Read the model definition and answer for the solid it produces. Units are mm, in the model's axes. Face numbers are marked on the shaded views. Give positions to 0.01 mm unless a question says otherwise; leave off trailing zeros. Order: outer loops, then holes, each group sorted by start corner. A loop starts at its lowest first (then second) coordinate and runs counter-clockwise, first axis right, second up. Notation, with made-up numbers: (-34, -36.5) -> (-8, -36.5) arc R18 cw to (-8, -5.5) -> close; hole circle Ø6 at (-30, -31.5). An arc over 180 degrees is marked (long way). One line per item, written item: value. Start each with the question number.
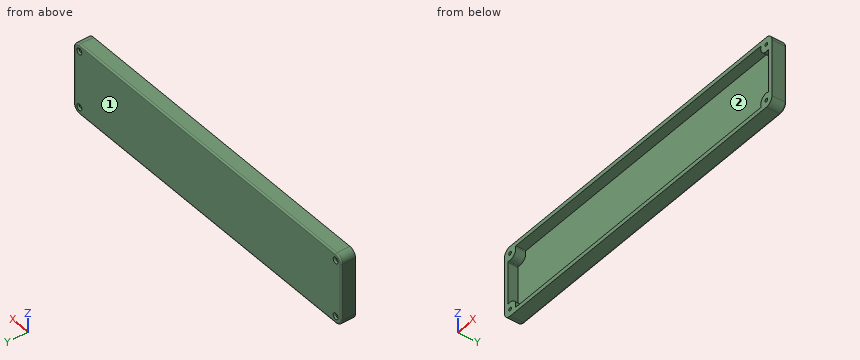
from build123d import *

# Parameters (mm, degrees)
BOSS_EXTRUDE1_DEPTH                                 = 10
CUT_EXTRUDE1_DEPTH                                  = 7
CSK_FOR_M2_COUNTERSUNK_FLAT_HEAD_SCREW2_D           = 2.4
CSK_FOR_M2_COUNTERSUNK_FLAT_HEAD_SCREW2_CSINK_D     = 4.4
CSK_FOR_M2_COUNTERSUNK_FLAT_HEAD_SCREW2_CSINK_ANGLE = 90
FILLET1_R                                           = 1


with BuildPart() as part:
    # Sketch1 → Boss-Extrude1 (new body)
    with BuildSketch(Plane(origin=(0, 0, 0), x_dir=(1, 0, 0), z_dir=(0, 1, 0))):
        with BuildLine():
            Line((-115, 25), (115, 25))
            ThreePointArc((115, 25), (118.535533906, 23.535533906), (120, 20))
            Line((120, 20), (120, -20))
            ThreePointArc((120, -20), (118.535533906, -23.535533906), (115, -25))
            Line((115, -25), (-115, -25))
            ThreePointArc((-115, -25), (-118.535533906, -23.535533906), (-120, -20))
            Line((-120, -20), (-120, 20))
            ThreePointArc((-120, 20), (-118.535533906, 23.535533906), (-115, 25))
        make_face()
    extrude(amount=-BOSS_EXTRUDE1_DEPTH)

    # Sketch2 → Cut-Extrude1 (cut)
    with BuildSketch(Plane.XZ.offset(10)):
        with BuildLine():
            ThreePointArc((110.125928985, 21.347074542), (111.23652041, 16.476032992), (115.978966674, 14.904516992))
            ThreePointArc((115.978966674, 14.904516992), (116.536912433, 15.216669336), (116.945654989, 14.725067791))
            Line((116.945654989, 14.725067791), (116.945654989, -14.725067791))
            ThreePointArc((116.945654989, -14.725067791), (116.58492435, -15.205280291), (116.023238809, -14.992583342))
            ThreePointArc((116.023238809, -14.992583342), (111.282334907, -16.506525423), (110.125928985, -21.347074542))
            ThreePointArc((110.125928985, -21.347074542), (110.043745309, -21.784949523), (109.644883292, -21.983438179))
            Line((109.644883292, -21.983438179), (-109.644883292, -21.983438179))
            ThreePointArc((-109.644883292, -21.983438179), (-110.043745309, -21.784949523), (-110.125928985, -21.347074542))
            ThreePointArc((-110.125928985, -21.347074542), (-111.42230579, -16.46889365), (-116.309291353, -15.206113484))
            ThreePointArc((-116.309291353, -15.206113484), (-116.747166334, -15.123929808), (-116.945654989, -14.725067791))
            Line((-116.945654989, -14.725067791), (-116.945654989, 14.725067791))
            ThreePointArc((-116.945654989, 14.725067791), (-116.746289712, 15.124590961), (-116.307179936, 15.205509941))
            ThreePointArc((-116.307179936, 15.205509941), (-111.411229141, 16.459961189), (-110.126182098, 21.347970622))
            ThreePointArc((-110.126182098, 21.347970622), (-110.043464387, 21.78532079), (-109.644883292, 21.983438179))
            Line((-109.644883292, 21.983438179), (109.644883292, 21.983438179))
            ThreePointArc((109.644883292, 21.983438179), (110.043745309, 21.784949523), (110.125928985, 21.347074542))
        make_face()
    extrude(amount=-CUT_EXTRUDE1_DEPTH, mode=Mode.SUBTRACT)

    # CSK for M2 Countersunk Flat Head Screw2 (through all)
    with Locations(Plane(origin=(-115, 0, -20), x_dir=(0, 0, 1), z_dir=(0, 1, 0))):
        with Locations((0, 0), (40, 0), (0, 230), (40, 230)):
            CounterSinkHole(CSK_FOR_M2_COUNTERSUNK_FLAT_HEAD_SCREW2_D / 2, CSK_FOR_M2_COUNTERSUNK_FLAT_HEAD_SCREW2_CSINK_D / 2, counter_sink_angle=CSK_FOR_M2_COUNTERSUNK_FLAT_HEAD_SCREW2_CSINK_ANGLE)

    # Fillet1
    fillet1_edges = [part.edges().sort_by_distance(p)[0] for p in [
        (-120, 0, 0),
        (-118.535533906, 0, -23.535533906),
        (0, 0, -25),
        (118.535533906, 0, -23.535533906),
        (120, 0, 0),
        (118.535533906, 0, 23.535533906),
        (0, 0, 25),
        (-118.535533906, 0, 23.535533906),
    ]]
    fillet(fillet1_edges, radius=FILLET1_R)


solid = part.part
Item 1: Find section C-C on y = -5.25. Write down the section's boundary in (x, z), then the cut area to 3 significant figures.
Item 2: Find section B-B on z = -5.5. Write down the section's boundary in (x, y), then the cut area to 3 significant figures.
Item 3: Find the intervals of material crossed by line 1 (X direction, y = -4.75, z = -20); line 2 (Z direction, x = 115, y = -4.5); line 3 (Z direction, x = -115, y = -7), in increasing order. Write a range as from..to.
Item 4: For a pull along Z with two mould halves and no side action, classify the marked faces 1 and 2 as +Z half, -Z half, draft (parallel to the pull), parting line (faces both ways), or undercut.
Item 5: Find section A-A on x = -21.5. Write down the section's boundary in (y, z), then the cut area to 3 significant figures.
Item 6: Flat-ended cylindrical pins translate along their axes: pin 1 (13 mm diameter, centred on x = -57.5, z = -3.5, fed in from -Y); pin 2 (3 mm diameter, centred on x = 115, z = -20, fed in from -Y); pin 3 (4 mm diameter, centred on x = -115, z = 20, fed in from +Y); pin 4 (1.4 mm diameter, centred on x = 115, z = 20, fed in from -Y). Find the tip coordinate at first contact, or state that the pin passes through.
Checks:
1. outline: (-120, -20) arc R5 ccw to (-115, -25) -> (115, -25) arc R5 ccw to (120, -20) -> (120, 20) arc R5 ccw to (115, 25) -> (-115, 25) arc R5 ccw to (-120, 20) -> close; hole (-116.95, -14.73) arc R0.5 ccw to (-116.31, -15.21) arc R5 cw to (-110.13, -21.35) arc R0.5 ccw to (-109.64, -21.98) -> (109.64, -21.98) arc R0.5 ccw to (110.13, -21.35) arc R5.06 cw to (116.02, -14.99) arc R0.5 ccw to (116.95, -14.73) -> (116.95, 14.73) arc R0.5 ccw to (115.98, 14.9) arc R5.09 cw to (110.13, 21.35) arc R0.5 ccw to (109.64, 21.98) -> (-109.64, 21.98) arc R0.5 ccw to (-110.13, 21.35) arc R4.99 cw to (-116.31, 15.21) arc R0.5 ccw to (-116.95, 14.73) -> close; hole circle Ø2.4 at (-115, -20); hole circle Ø2.4 at (-115, 20); hole circle Ø2.4 at (115, -20); hole circle Ø2.4 at (115, 20)
1. area: 1,850 mm2
2. outline: (-120, -10) -> (-116.95, -10) -> (-116.95, -3) -> (116.95, -3) -> (116.95, -10) -> (120, -10) -> (120, -1) arc R1 ccw to (119, 0) -> (-119, 0) arc R1 ccw to (-120, -1) -> close
2. area: 762 mm2
3. line 1: -120..-116.2, -113.8..-109.95, 109.93..113.8, 116.2..120
3. line 2: -25..-21.2, -18.8..-14.89, 14.81..18.8, 21.2..25
3. line 3: -25..-21.2, -18.8..-15.02, 15.01..18.8, 21.2..25
4. face 1: draft
4. face 2: undercut
5. outline: (-10, -25) -> (-1, -25) arc R1 ccw to (0, -24) -> (0, 24) arc R1 ccw to (-1, 25) -> (-10, 25) -> (-10, 21.98) -> (-3, 21.98) -> (-3, -21.98) -> (-10, -21.98) -> close
5. area: 192 mm2
6. pin 1: y = -3
6. pin 2: y = -10
6. pin 3: y = -0.2
6. pin 4: through
